```python
from build123d import *

# Parameters (mm, degrees)
BOSS_EXTRUDE1_START = -2
SKETCH1_R           = 0.8
BOSS_EXTRUDE1_DEPTH = 1.5


with BuildPart() as part:
    # Sketch1 → Boss-Extrude1 (new body)
    with BuildSketch(Plane.XY.offset(BOSS_EXTRUDE1_START)):
        with BuildLine():
            Line((-9.740911438, -2.722813484), (-8.476189779, -5.495368755))
            Line((-8.476189779, -5.495368755), (-4.334626233, -3.606163814))
            add(Edge.make_bspline(
                [(-4.334626233, -3.606163814), (-4.220059154, -3.746893984), (-4.098911696, -3.882323382), (-3.971959366, -4.012075441)],
                knots=[0, 0, 0, 0, 0.126750823, 0.126750823, 0.126750823, 0.126750823], degree=3))
            add(Edge.make_bspline(
                [(4.494162658, -3.699077527), (3.751409152, -4.48949841), (0.818181256, -5.496970155), (-2.253055886, -4.873398081), (-3.971959366, -4.012075441)],
                knots=[0, 0, 0, 0, 0.35390124, 1, 1, 1, 1], degree=3))
            Line((4.494162658, -3.699077527), (8.498351825, -5.462813486))
            Line((8.498351825, -5.462813486), (9.73228444, -2.722813484))
            Line((9.73228444, -2.722813484), (7.667616443, -1.793010133))
            Line((7.667616443, -1.793010133), (7.696555299, -1.640039759))
            add(Edge.make_bspline(
                [(6.39631974, 5.064495713), (6.677952564, 4.488955557), (7.263392082, 3.091949217), (7.791107632, 0.878451291), (7.813586585, -0.798840627), (7.703296692, -1.594388982), (7.696555299, -1.640039759)],
                knots=[0.013511716, 0.013511716, 0.013511716, 0.013511716, 0.127684465, 0.281511893, 0.415370359, 0.42352788, 0.42352788, 0.42352788, 0.42352788], degree=3))
            Line((6.39631974, 5.064495713), (-6.412751764, 5.064495713))
            add(Edge.make_bspline(
                [(-7.706044999, -1.640039759), (-7.92409566, -0.185434038), (-7.675413336, 2.149266822), (-6.7968854, 4.310558244), (-6.412751764, 5.064495713)],
                knots=[0, 0, 0, 0, 0.611703094, 0.967799176, 0.967799176, 0.967799176, 0.967799176], degree=3))
            Line((-7.706044999, -1.640039759), (-7.676243441, -1.793010133))
            Line((-7.676243441, -1.793010133), (-9.740911438, -2.722813484))
        make_face()
        with Locations((-8.091798032, -3.657959287)):
            Circle(SKETCH1_R, mode=Mode.SUBTRACT)
        with Locations((7.909888927, -3.569882761)):
            Circle(SKETCH1_R, mode=Mode.SUBTRACT)
    extrude(amount=-BOSS_EXTRUDE1_DEPTH)


solid = part.part
```
Input: part model. Units: mm. Frame: model coordinates. A direction names the side the tool comes from. Round coordinates to 2 decimals unless told otherwise and drop trailing zeros. Loops run counter-clockwise (first coordinate to the right, second up) from the corner with the lowest first, then second, coordinate; pieces in that order, holes last. Notation, with made-up numbers: (-5, 68) -> (24, 68) arc R23 ccw to (24, 97) -> close; hole circle Ø3 at (48, 15.5). An arc over 180 degrees is marked (long way). One line per item, written item: value.
(1) Set-up query: faces 4 (the face through (-6.43, -4.56, -2.74)), 5 (the face through (0, 5.064, -3)). Return all of +Z, -Z, +X, -X, +Y, -Y with unobstructed straight access to the full face (end or side cutting, diameter ignored); none if empty.
Geometry check:
face 4: +Z, -Z, -Y
face 5: +Z, -Z, +X, -X, +Y
(2) Section A-A (z = -2.3). Give the number of separate pieces and of enclosed holes in the cut face, plus the area to 3 significant figures.
Geometry check:
separate pieces: 1
enclosed holes: 2
area: 150 mm2
(3) Mould query, pull axis X, two halves, no side actions, for faces 1 (the face through (-7.33, -3.42, -2.74)), 2 (the face through (9.107, -4.112, -2.74)), 3 (the face through (0, 0, -3.5)). Classes: pulls with the +X half, pulls with the -X half, needs draft (parallel to the pull), parting line crosses it, or undercut.
Geometry check:
face 1: undercut
face 2: pulls with the +X half
face 3: needs draft
(4) Section B-B (x = 4.75). Return the cut outline in (y, z).
Geometry check:
outline: (-3.81, -3.5) -> (5.06, -3.5) -> (5.06, -2) -> (-3.81, -2) -> close
(5) Material intervals for line 1 (X direction, y = -3.25, z = -3.05); line 2 (Y direction, x = 0.25, z = -2.45); line 3 (X direction, y = 0.5, z = -2.7), sorted ascending. Write a range as [from, to].
Geometry check:
line 1: [-9.5, -8.78], [-7.4, 7.18], [8.64, 9.49]
line 2: [-5.08, 5.06]
line 3: [-7.77, 7.74]
